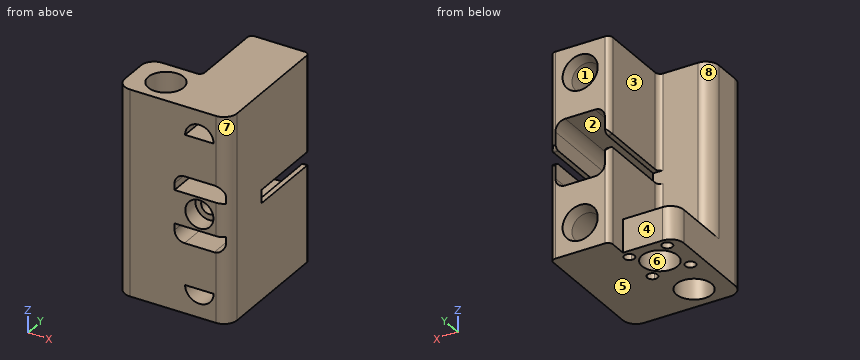
from build123d import *

# Parameters (mm, degrees)
F0_W            = 18
F0_H            = 62
F0_R            = 4.315
F1_DEPTH        = 40
F3_DEPTH        = 16
F4_R            = 5.35
F5_DEPTH        = 100
F6_R            = 1.5625
F6_R_2          = 5.375
F7_DEPTH        = 10
F8_DEPTH        = 10
F10_DEPTH       = 100
F9_W            = 1.5
F9_H            = 2
F11_DEPTH       = 24
F12_W           = 15
F12_H           = 10
F13_DEPTH       = 8
F14_SIZE2       = 3
F14_SIZE        = 1
F14_2_SIZE2     = 3
F14_2_SIZE      = 1
F15_R           = 3
F16_T1_DEPTH    = 62
F16_T3_DEPTH    = 82
F16_T5_DEPTH    = 30
F17_R           = 1.49999
F18_D           = 5
F18_DEPTH       = 10
F18_CBORE_D     = 8.5
F18_CBORE_DEPTH = 5
F18_TIP         = 1.5021515476


# Not quite as in the source:
# - a fillet or chamfer that OpenCascade refuses, or shapes differently, is made with other operations: its cross-section is extruded or revolved along the edge and cut away or added
# - a fillet or chamfer is up to 0.001 mm smaller than in the source, because OpenCascade refuses the exact size


with BuildPart() as f1:
    # F0 (on Front) → F1 (new body)
    with BuildSketch(Plane.XZ):
        Rectangle(F0_W, F0_H)
        with Locations((0, -22.5)):
            Circle(F0_R, mode=Mode.SUBTRACT)
        with Locations((0, 22.5)):
            Circle(F0_R, mode=Mode.SUBTRACT)
    extrude(amount=F1_DEPTH)

    # F2 (on face) → F3 (join)
    with BuildSketch(Plane(origin=(-9, 0, 0), x_dir=(0, -1, 0), z_dir=(-1, 0, 0))):
        Polygon((24, 31), (24, 0), (24, -31), (40, -31), (40, 31), align=None)
    extrude(amount=F3_DEPTH)

    # F4 (on face) → F5 (cut)
    with BuildSketch(Plane(origin=(0, 0, -31), x_dir=(1, 0, 0), z_dir=(0, 0, -1))):
        with Locations((-15, 32)):
            Circle(F4_R)
    extrude(amount=-F5_DEPTH, mode=Mode.SUBTRACT)

    # F6 (on face) → F7 (join)
    with BuildSketch(Plane(origin=(0, 0, -31), x_dir=(1, 0, 0), z_dir=(0, 0, -1))):
        with BuildLine():
            Line((-9, 22.2923703349), (-9, 24))
            Line((-9, 24), (-25, 24))
            Line((-25, 24), (-25, 6.5))
            Line((-25, 6.5), (-9, 6.5))
            Line((-9, 6.5), (-9, 7.7076296651))
            ThreePointArc((-9, 7.7076296651), (-10.8125, 9.25), (-9, 10.7923703349))
            Line((-9, 10.7923703349), (-9, 19.2076296651))
            ThreePointArc((-9, 19.2076296651), (-10.8125, 20.75), (-9, 22.2923703349))
        make_face()
        with Locations((-20.75, 9.25)):
            Circle(F6_R, mode=Mode.SUBTRACT)
        with Locations((-15, 15)):
            Circle(F6_R_2, mode=Mode.SUBTRACT)
        with Locations((-20.75, 20.75)):
            Circle(F6_R, mode=Mode.SUBTRACT)
    extrude(amount=-F7_DEPTH)

    # F6 (on face) → F8 (cut)
    with BuildSketch(Plane(origin=(0, 0, -31), x_dir=(1, 0, 0), z_dir=(0, 0, -1))):
        with BuildLine():
            ThreePointArc((-7.6875, 20.75), (-8.0600354522, 21.7626157341), (-9, 22.2923703349))
            Line((-9, 22.2923703349), (-9, 19.2076296651))
            ThreePointArc((-9, 19.2076296651), (-8.0600354522, 19.7373842659), (-7.6875, 20.75))
        make_face()
        with BuildLine():
            ThreePointArc((-7.6875, 9.25), (-8.0600354522, 10.2626157341), (-9, 10.7923703349))
            Line((-9, 10.7923703349), (-9, 7.7076296651))
            ThreePointArc((-9, 7.7076296651), (-8.0600354522, 8.2373842659), (-7.6875, 9.25))
        make_face()
    extrude(amount=-F8_DEPTH, mode=Mode.SUBTRACT)

    # F9 (on face) → F10 (cut)
    with BuildSketch(Plane(origin=(0, 0, 0), x_dir=(-1, 0, 0), z_dir=(0, 1, 0))):
        Polygon((7.5, 2), (7.5, 10), (-7.5, 10), (-7.5, 2), (-7.5, 0), (0, 0), (7.5, 0), align=None)
        Polygon((7.5, -2), (7.5, 0), (0, 0), (-7.5, 0), (-7.5, -2), (-7.5, -10), (7.5, -10), align=None)
    extrude(amount=-F10_DEPTH, mode=Mode.SUBTRACT)

    # F9 (on face) → F11 (cut)
    with BuildSketch(Plane(origin=(0, 0, 0), x_dir=(-1, 0, 0), z_dir=(0, 1, 0))):
        with Locations((-8.25, -1)):
            Rectangle(F9_W, F9_H)
        with Locations((-8.25, 1)):
            Rectangle(F9_W, F9_H)
        with Locations((8.25, -1)):
            Rectangle(F9_W, F9_H)
        with Locations((8.25, 1)):
            Rectangle(F9_W, F9_H)
    extrude(amount=-F11_DEPTH, mode=Mode.SUBTRACT)

    # F12 (on face) → F13 (join)
    with BuildSketch(Plane.XZ.offset(40)):
        Rectangle(F12_W, F12_H)
        with BuildLine():
            Line((4.315, 22.5), (0, 22.5))
            Line((0, 22.5), (-4.315, 22.5))
            ThreePointArc((-4.315, 22.5), (0, 18.185), (4.315, 22.5))
        make_face()
        with BuildLine():
            Line((-4.315, -22.5), (0, -22.5))
            Line((0, -22.5), (4.315, -22.5))
            ThreePointArc((4.315, -22.5), (0, -18.185), (-4.315, -22.5))
        make_face()
    extrude(amount=-F13_DEPTH)

    # F14
    f14_edges = [f1.edges().sort_by_distance(p)[0] for p in [
        (-4.315, 0, 22.5),
    ]]
    f14_side = f1.faces().sort_by_distance((8.25, 0, 2.341321))[0]
    chamfer(f14_edges, length=F14_SIZE, length2=F14_SIZE2, reference=f14_side)

    # F14#2
    f14_2_edges = [f1.edges().sort_by_distance(p)[0] for p in [
        (-4.315, 0, -22.5),
    ]]
    f14_2_side = f1.faces().sort_by_distance((0, 0, -30.658679))[0]
    chamfer(f14_2_edges, length=F14_2_SIZE, length2=F14_2_SIZE2, reference=f14_2_side)

    # F15
    f15_edges = [f1.edges().sort_by_distance(p)[0] for p in [
        (-7.5, -20, 10),
        (7.5, -20, 10),
        (7.5, -20, -10),
        (-7.5, -20, -10),
    ]]
    fillet(f15_edges, radius=F15_R)

    # F16: fillet of radius 4 on 4 edges, made by hand

    # F16_s2 → F16_t1 (cut)
    with BuildSketch(Plane.XY.offset(-21)):
        with BuildLine():
            ThreePointArc((-21, -24), (-23.8284271247, -25.1715728753), (-25, -28))
            Line((-25, -28), (-25, -24))
            Line((-25, -24), (-21, -24))
        make_face()
    extrude(amount=F16_T1_DEPTH, mode=Mode.SUBTRACT)

    # F16_s4 → F16_t3 (cut)
    with BuildSketch(Plane.XY.offset(-41)):
        with BuildLine():
            ThreePointArc((-21, -40), (-23.8284271247, -38.8284271247), (-25, -36))
            Line((-25, -36), (-25, -40))
            Line((-25, -40), (-21, -40))
        make_face()
        with BuildLine():
            ThreePointArc((9, -36), (7.8284271247, -38.8284271247), (5, -40))
            Line((5, -40), (9, -40))
            Line((9, -40), (9, -36))
        make_face()
    extrude(amount=F16_T3_DEPTH, mode=Mode.SUBTRACT)

    # F16_s6 → F16_t5 (cut)
    with BuildSketch(Plane.XY.offset(-41)):
        with BuildLine():
            ThreePointArc((-21, -6.5), (-23.8284271247, -7.6715728753), (-25, -10.5))
            Line((-25, -10.5), (-25, -6.5))
            Line((-25, -6.5), (-21, -6.5))
        make_face()
    extrude(amount=F16_T5_DEPTH, mode=Mode.SUBTRACT)

    # F17 (radius 1.5 in the source; OpenCascade refuses exactly that, so slightly less here)
    f17_edges = [f1.edges().sort_by_distance(p)[0] for p in [
        (-25, -10.5, -26),
        (-9, 0, -16.5),
        (9, 0, -16.5),
        (-9, -24, -11.5),
        (-9, -24, 16.5),
        (9, 0, 16.5),
        (-9, 0, 16.5),
        (-8.25, 0, 2),
        (-8.25, 0, -2),
        (8.25, 0, -2),
        (8.25, 0, 2),
    ]]
    fillet(f17_edges, radius=F17_R)

    # F18
    with Locations(Plane.XZ.offset(40)):
        with Locations((0, 0)):
            CounterBoreHole(F18_D / 2, F18_CBORE_D / 2, F18_CBORE_DEPTH, depth=F18_DEPTH)
            with Locations((0, 0, -(F18_DEPTH + F18_TIP / 2))):  # 118° drill point
                Cone(0, F18_D / 2, F18_TIP, mode=Mode.SUBTRACT)


solid = f1.part
Verification items for the finished model (mm, model axes). Face numbers are marked on the shaded views. A direction names the side the tool comes from. Give positions to 0.01 mm unless a question says otherwise; leave off trailing zeros. Loops run counter-clockwise (first coordinate to the right, second up) from the corner with the lowest first, then second, coordinate; pieces in that order, holes last.
1) Sectioned sample at A-A, the plane z = 0. Enter the section's corners in (x, y).
2) Sectioned sample at C-C, the plane x = 0. Count the separate pieces of the cut face and the enclosed holes in it, then the cut area to 3 significant figures.
3) Depth check by flat-ended pin: pin 1 Ø3 at (x, z) = (-17.5, 9.5) entering from +Y; pin 2 Ø11 at (y, z) = (-20, -3.5) entering from -X; pin 3 Ø14 at (x, y) = (-15, -15) entering from -Z; pin 4 Ø5 at (x, z) = (-10, -2) entering from +Y. Enter the tip coordinate at first touch or a pass-through.
4) Thickness scan on line 1 along Y through (x, z) = (-9.25, -23.25); line 2 along X through (y, z) = (-32, -17); line 3 along X through (y, z) = (-22.5, -6.5). Record the ranges inside material, lowest first.
5) Sectioned sample at B-B, the plane y = -15. Enter the section's corners in (x, z) (3 decimals), then the cut area to 3 significant figures.
6) Draft check along Y on the marked faces 5, 6, 7 and 8. Enter one of: pulls with the +Y half, pulls with the -Y half, needs draft (parallel to the pull), parting line crosses it, or undercut.
7) Set-up check for the marked faces 1, 2, 3 and 4: record each of +Z, -Z, +X, -X, +Y, -Y from which the full face is reachable in a straight line by a thin tool's end or side.
Answers:
1. outline: (-25, -36) arc R4 ccw to (-21, -40) - (-4.25, -40) - (-4.25, -35) - (-2.5, -35) - (-2.5, -32) - (-7.5, -32) - (-7.5, -24) - (-21, -24) arc R4 ccw to (-25, -28) - close; (2.5, -35) - (4.25, -35) - (4.25, -40) - (5, -40) arc R4 ccw to (9, -36) - (9, -24) - (7.5, -24) - (7.5, -32) - (2.5, -32) - close; hole circle Ø10.7 at (-15, -32)
2. separate pieces: 6
2. enclosed holes: 0
2. area: 1,080 mm2
3. pin 1: stops at y = -24
3. pin 2: stops at x = -24.12
3. pin 3: stops at z = -31
3. pin 4: stops at y = -0.03
4. line 1: y = -40 to -22.31, -19.19 to -10.81, -7.69 to -6.5
4. line 2: x = -25 to -20.35, -9.65 to 9
4. line 3: x = -9 to -7.5, 7.5 to 9
5. outline: (-25, -31) - (-20.375, -31) - (-20.375, -21) - (-25, -21) - close; (-9.625, -31) - (9, -31) - (9, -2) - (7.5, -2) - (7.5, -7) arc R3 cw to (4.5, -10) - (-4.5, -10) arc R3 cw to (-7.5, -7) - (-7.5, -2) - (-9, -2) - (-9, -21) - (-9.625, -21) - close; (-9, 2) - (-7.5, 2) - (-7.5, 7) arc R3 cw to (-4.5, 10) - (4.5, 10) arc R3 cw to (7.5, 7) - (7.5, 2) - (9, 2) - (9, 31) - (-9, 31) - close; hole circle Ø8.63 at (0, -22.5); hole circle Ø8.63 at (0, 22.5)
5. area: 747 mm2
6. face 5: needs draft
6. face 6: undercut
6. face 7: pulls with the -Y half
6. face 8: pulls with the +Y half
7. face 1: +Y
7. face 2: +Y, -Y
7. face 3: +Z, -X, +Y
7. face 4: +Z, -Z, -X, +Y
